```python
from build123d import *

# Parameters (mm, degrees)
F0_R     = 28
F1_DEPTH = 25
F2_W     = 4.0792156109
F2_H     = 4.4
F3_DEPTH = 30
F4_R     = 5
F4_R_2   = 3.5
F5_DEPTH = 1


# Not quite as in the source:
# - ends of sketch curves that miss each other by under 0.0002 mm in the source are joined


with BuildPart() as f1:
    # F0 (on Top) → F1 (new body)
    with BuildSketch(Plane.XY):
        Circle(F0_R)
        with BuildLine():
            ThreePointArc((22.6064085074, 10.6747503202), (24.3942638, 5.4699080119), (25, 0))
            ThreePointArc((25, 0), (24.6306042082, -4.2817445441), (23.5333330927, -8.4369564149))
            ThreePointArc((23.5333330927, -8.4369564149), (21.1171584026, -13.3815403074), (17.6776695297, -17.6776695297))
            ThreePointArc((17.6776695297, -17.6776695297), (14.3888166579, -20.4441178628), (10.6747503202, -22.6064085074))
            ThreePointArc((10.6747503202, -22.6064085074), (5.4699080119, -24.3942638), (0, -25))
            ThreePointArc((0, -25), (-4.2817445441, -24.6306042082), (-8.4369564149, -23.5333330927))
            ThreePointArc((-8.4369564149, -23.5333330927), (-13.3815403074, -21.1171584026), (-17.6776695297, -17.6776695297))
            ThreePointArc((-17.6776695297, -17.6776695297), (-20.4441178628, -14.3888166579), (-22.6064085074, -10.6747503202))
            ThreePointArc((-22.6064085074, -10.6747503202), (-24.3942638, -5.4699080119), (-25, 0))
            ThreePointArc((-25, 0), (-24.6306042082, 4.2817445441), (-23.5333330927, 8.4369564149))
            ThreePointArc((-23.5333330927, 8.4369564149), (-21.1171584026, 13.3815403074), (-17.6776695297, 17.6776695297))
            ThreePointArc((-17.6776695297, 17.6776695297), (-14.3888166579, 20.4441178628), (-10.6747503202, 22.6064085074))
            ThreePointArc((-10.6747503202, 22.6064085074), (-5.4699080119, 24.3942638), (0, 25))
            ThreePointArc((0, 25), (4.2817445441, 24.6306042082), (8.4369564149, 23.5333330927))
            ThreePointArc((8.4369564149, 23.5333330927), (13.3815403074, 21.1171584026), (17.6776695297, 17.6776695297))
            ThreePointArc((17.6776695297, 17.6776695297), (20.4441178628, 14.3888166579), (22.6064085074, 10.6747503202))
        make_face(mode=Mode.SUBTRACT)
        with BuildLine():
            ThreePointArc((23.5333330927, -8.4369564149), (24.6306042082, -4.2817445441), (25, 0))
            ThreePointArc((25, 0), (15.0015557257, -9.999999879), (5.0000004841, -0.0031114513))
            ThreePointArc((5.0000004841, -0.0031114513), (16.8293380679, 0.3461163718), (22.6064085074, 10.6747503202))
            ThreePointArc((22.6064085074, 10.6747503202), (20.4441178628, 14.3888166579), (17.6776695297, 17.6776695297))
            ThreePointArc((17.6776695297, 17.6776695297), (17.6787695083, 3.5366340557), (3.5377343766, 3.5333341199))
            ThreePointArc((3.5377343766, 3.5333341199), (11.6553978371, 12.1448803043), (8.4369564149, 23.5333330927))
            ThreePointArc((8.4369564149, 23.5333330927), (4.2817445441, 24.6306042082), (0, 25))
            ThreePointArc((0, 25), (9.999999879, 15.0015557257), (0.0031114513, 5.0000004841))
            ThreePointArc((0.0031114513, 5.0000004841), (-0.3461163718, 16.8293380679), (-10.6747503202, 22.6064085074))
            ThreePointArc((-10.6747503202, 22.6064085074), (-14.3888166579, 20.4441178628), (-17.6776695297, 17.6776695297))
            ThreePointArc((-17.6776695297, 17.6776695297), (-3.5366340557, 17.6787695083), (-3.5333341199, 3.5377343766))
            ThreePointArc((-3.5333341199, 3.5377343766), (-12.1448803043, 11.6553978371), (-23.5333330927, 8.4369564149))
            ThreePointArc((-23.5333330927, 8.4369564149), (-24.6306042082, 4.2817445441), (-25, 0))
            ThreePointArc((-25, 0), (-15.0015556407, 9.999999879), (-5.000000484, 0.0031112813))
            ThreePointArc((-5.000000484, 0.0031112813), (-16.8293380679, -0.3461163718), (-22.6064085074, -10.6747503202))
            ThreePointArc((-22.6064085074, -10.6747503202), (-20.4441178628, -14.3888166579), (-17.6776695297, -17.6776695297))
            ThreePointArc((-17.6776695297, -17.6776695297), (-17.6787695083, -3.5366340557), (-3.5377343766, -3.5333341199))
            ThreePointArc((-3.5377343766, -3.5333341199), (-11.6553978371, -12.1448803043), (-8.4369564149, -23.5333330927))
            ThreePointArc((-8.4369564149, -23.5333330927), (-4.2817445441, -24.6306042082), (0, -25))
            ThreePointArc((0, -25), (-9.999999879, -15.0015557257), (-0.0031114513, -5.0000004841))
            ThreePointArc((-0.0031114513, -5.0000004841), (0.3461163718, -16.8293380679), (10.6747503202, -22.6064085074))
            ThreePointArc((10.6747503202, -22.6064085074), (14.3888166579, -20.4441178628), (17.6776695297, -17.6776695297))
            ThreePointArc((17.6776695297, -17.6776695297), (3.5366340557, -17.6787695083), (3.5333341199, -3.5377343766))
            ThreePointArc((3.5333341199, -3.5377343766), (12.1448803043, -11.6553978371), (23.5333330927, -8.4369564149))
        make_face()
    extrude(amount=F1_DEPTH)

    # F2 (on Top) → F3 (cut)
    with BuildSketch(Plane.XY):
        with BuildLine():
            Line((-2.0396078054, -2.2), (-2.0396078054, 2.2))
            ThreePointArc((-2.0396078054, 2.2), (-3, 0), (-2.0396078054, -2.2))
        make_face()
        Rectangle(F2_W, F2_H)
        with BuildLine():
            ThreePointArc((2.0396078054, -2.2), (2.7494384351, -1.2002450966), (3, 0))
            ThreePointArc((3, 0), (2.7494384351, 1.2002450966), (2.0396078054, 2.2))
            Line((2.0396078054, 2.2), (2.0396078054, -2.2))
        make_face()
    extrude(amount=F3_DEPTH, mode=Mode.SUBTRACT)

    # F4 (on Top) → F5 (join)
    with BuildSketch(Plane.XY):
        Circle(F4_R)
        Circle(F4_R_2, mode=Mode.SUBTRACT)
    extrude(amount=-F5_DEPTH)


solid = f1.part
```
Check sheet for the modelled part. Datum: model origin and axes. Units: mm. A direction names the side the tool comes from. Coordinates: 2 decimals unless noted, no trailing zeros. Write each loop counter-clockwise with the first axis right and the second up, starting at its lowest first coordinate (ties: lowest second). Pieces come first, ordered by that corner, then holes. Notation, with made-up numbers: M 39.25,-22.5 L 43.25,-22.5 A10 ccw 43.25,-8.5 Z; hole C 65,35.5 d11. An arc over 180 degrees is marked long. Use one line per item in the form item = value.
Item 1: Release check for a two-part mould opening along Y. For faces 1 (the face through (0, -2.2, 12)), 2 (the face through (6, 0, 0)) record: pulls with the +Y half, pulls with the -Y half, needs draft (parallel to the pull), parting line crosses it, or undercut.
Answer below:
face_1 = undercut
face_2 = needs draft
Item 2: Material ranges on L1, parallel to Y at x = 0, z = -0.8; L2, parallel to Y at x = -12.5, z = 21.75; L3, parallel to Y at x = -15.5, z = 6, recorded low to high. Write a range as from..to.
Answer below:
L1 = -5..-3.5, 3.5..5
L2 = -25.05..-21.65, -0.79..1.24, 9.68..11.74, 20.43..25.05
L3 = -23.32..-19.62, -1.89..0.35, 9.99..11.99, 19.33..23.32
Item 3: Gauge pin test, flat ends, axial feed: pin 1 Ø4 at (y, z) = (18, 9.5) entering from -X; pin 2 Ø12 at (y, z) = (-17.5, 9) entering from -X; pin 3 Ø4 at (x, y) = (0, 0) entering from -Z; pin 4 Ø5 at (x, z) = (6, 18.5) entering from -Y. Record the tip position at first contact, or that the pin passes through.
Answer below:
pin_1 = -22.98
pin_2 = -25.53
pin_3 = through
pin_4 = -27.78
Item 4: Sectioned sample at B-B, the plane z = 19.5. State how many separate pieces and enclosed holes the cut face has, and give its area (3 significant figures).
Answer below:
separate_pieces = 1
enclosed_holes = 9
area = 974 mm^2
Item 5: Set-up check for faces 3 (the face through (0, 2.4, 0)), 4 (the face through (0, 2.2, 12)), 5 (the face through (6, 0, 25)): record each of +Z, -Z, +X, -X, +Y, -Y from which the full face is reachable in a straight line by a thin tool's end or side.
Answer below:
face_3 = -Z
face_4 = +Z, -Z
face_5 = +Z, +X, -X, +Y, -Y
Item 6: Sectioned sample at D-D, the plane y = 6.5. Record the cut outline in (x, z).
Answer below:
outline = M -27.24,0 L -22.6,0 L -22.6,25 L -27.24,25 Z; M -7.4,0 L -4.91,0 L -4.91,25 L -7.4,25 Z; M -1.49,0 L 0.67,0 L 0.67,25 L -1.49,25 Z; M 5.27,0 L 8.47,0 L 8.47,25 L 5.27,25 Z; M 19.72,0 L 21.88,0 L 21.88,25 L 19.72,25 Z; M 24.14,0 L 27.24,0 L 27.24,25 L 24.14,25 Z
Item 7: Sectioned sample at A-A, the plane x = -15. Record the cut outline in (y, z).
Answer below:
outline = M -23.64,0 L -20,0 L -20,25 L -23.64,25 Z; M -1.62,0 L 0.56,0 L 0.56,25 L -1.62,25 Z; M 10,0 L 12,0 L 12,25 L 10,25 Z; M 19.59,0 L 23.64,0 L 23.64,25 L 19.59,25 Z
